Verification items for the finished model (mm, model axes). Face numbers are marked on the shaded views. A direction names the side the tool comes from. Coordinates: 2 decimals unless noted, no trailing zeros. Order: outer loops, then holes, each group sorted by start corner. A loop starts at its lowest first (then second) coordinate and runs counter-clockwise, first axis right, second up. Notation, with made-up numbers: M 53.5,-25.5 L 92.5,-25.5 A24 cw 92.5,-1.5 Z; hole C 57,-21.5 d2. An arc over 180 degrees is marked long. Return JSON: item names as keys, results as strings. Group by question number.
Q1. Section check C-C, the plane x = 33.8. Enter the section's corners in (y, z), then the cut area to 3 significant figures.
Q2. Thickness scan on probe 1 along Y at (x, z) = (33.8, 12); probe 2 along X at (y, z) = (64.8, 6.5); probe 3 along Y at (x, z) = (10, 4.25). Record the ranges inside material, lowest first.
Q3. Section check A-A, the plane z = 13.25. Count the separate pieces of the cut face and the enclosed holes in it, then the cut area to 3 significant figures.
Q4. Go/stop test with flat-tipped pins: pin 1 Ø4 at (x, y) = (25, 21.5) entering from -Z; pin 2 Ø5 at (x, y) = (9.5, 39.5) entering from +Z; pin 3 Ø1.3 at (x, y) = (10.5, 3.5) entering from +Z; pin 4 Ø2.5 at (x, z) = (17.5, 6) entering from +Y. Record where each tip stops, or that it passes through.
Q5. Section check B-B, the plane y = 48. Enter the section's corners in (x, z), then the cut area to 3 significant figures.
Q6. Access from +Z, -Z, +X, -X, +Y, -Y to the whole of each face (thin tool, end or side, straight path). Record for the marked faces 1, 2, 3, 4 and 5.
from build123d import *

# Parameters (mm, degrees)
SKETCH_W      = 36
SKETCH_H      = 67
PAD_DEPTH     = 2
SKETCH002_W   = 1.5
SKETCH002_H   = 22
SKETCH002_W_2 = 6
SKETCH002_H_2 = 1.5
PAD001_DEPTH  = 12.75
SKETCH001_W   = 21
SKETCH001_H   = 15
SKETCH001_R   = 0.8
PAD006_DEPTH  = 8
SKETCH018_W   = 4.4
SKETCH018_H   = 4.4
SKETCH018_R   = 0.8
PAD020_DEPTH  = 13.75


with BuildPart() as part:
    # Sketch → Pad (new body)
    with BuildSketch(Plane.XY):
        with Locations((18, 33.5)):
            Rectangle(SKETCH_W, SKETCH_H)
    extrude(amount=PAD_DEPTH)

    # Sketch002 (on DatumPlane) → Pad001 (join)
    with BuildSketch(Plane.XY.offset(2)):
        with Locations((10.25, 39.5)):
            Rectangle(SKETCH002_W, SKETCH002_H)
        with Locations((18, 29.25)):
            Rectangle(SKETCH002_W_2, SKETCH002_H_2)
        with Locations((25.75, 39.5)):
            Rectangle(SKETCH002_W, SKETCH002_H)
        with Locations((18, 49.75)):
            Rectangle(SKETCH002_W_2, SKETCH002_H_2)
    extrude(amount=PAD001_DEPTH)

    # Sketch001 (on DatumPlane) → Pad006 (join)
    with BuildSketch(Plane.XY.offset(2)):
        with Locations((18, 7.5)):
            Rectangle(SKETCH001_W, SKETCH001_H)
        with Locations((10.253, 3.69)):
            Circle(SKETCH001_R, mode=Mode.SUBTRACT)
        with Locations((25.747, 3.69)):
            Circle(SKETCH001_R, mode=Mode.SUBTRACT)
    extrude(amount=PAD006_DEPTH)

    # Sketch018 (on DatumPlane) → Pad020 (join)
    with BuildSketch(Plane.XY.offset(2)):
        with Locations((2.2, 2.2)):
            Rectangle(SKETCH018_W, SKETCH018_H)
        with Locations((2.2, 2.2)):
            Circle(SKETCH018_R, mode=Mode.SUBTRACT)
        with Locations((33.8, 2.2)):
            Rectangle(SKETCH018_W, SKETCH018_H)
        with Locations((33.8, 2.2)):
            Circle(SKETCH018_R, mode=Mode.SUBTRACT)
        with Locations((33.8, 64.8)):
            Rectangle(SKETCH018_W, SKETCH018_H)
        with Locations((33.8, 64.8)):
            Circle(SKETCH018_R, mode=Mode.SUBTRACT)
        with Locations((2.2, 64.8)):
            Rectangle(SKETCH018_W, SKETCH018_H)
        with Locations((2.2, 64.8)):
            Circle(SKETCH018_R, mode=Mode.SUBTRACT)
    extrude(amount=PAD020_DEPTH)


solid = part.part
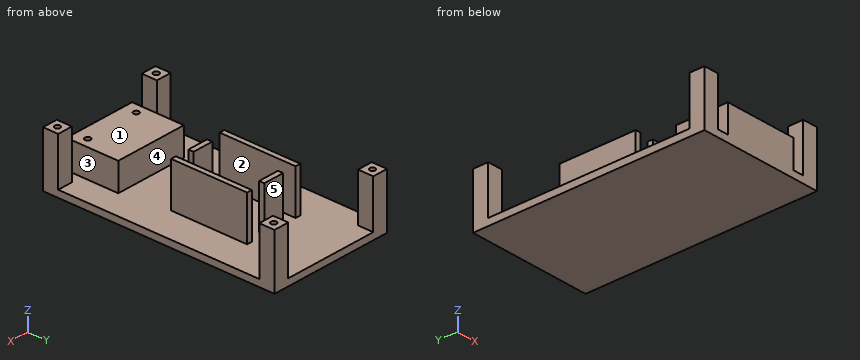
Numbers:
{
 "1": {"outline": "M 0,0 L 67,0 L 67,15.75 L 65.6,15.75 L 65.6,2 L 64,2 L 64,15.75 L 62.6,15.75 L 62.6,2 L 4.4,2 L 4.4,15.75 L 3,15.75 L 3,2 L 1.4,2 L 1.4,15.75 L 0,15.75 Z", "area": "211 mm2"},
 "2": {"probe 1": "y = 0 to 1.4, 3 to 4.4, 62.6 to 64, 65.6 to 67", "probe 2": "x = 0 to 1.4, 3 to 4.4, 31.6 to 33, 34.6 to 36", "probe 3": "y = 0 to 2.93, 4.45 to 15, 28.5 to 50.5"},
 "3": {"separate pieces": "8", "enclosed holes": "4", "area": "153 mm2"},
 "4": {"pin 1": "stops at z = 0", "pin 2": "stops at z = 14.75", "pin 3": "stops at z = 10", "pin 4": "stops at y = 50.5"},
 "5": {"outline": "M 0,0 L 36,0 L 36,2 L 26.5,2 L 26.5,14.75 L 25,14.75 L 25,2 L 11,2 L 11,14.75 L 9.5,14.75 L 9.5,2 L 0,2 Z", "area": "110 mm2"},
 "6": {"face 1": "+Z, -Y", "face 2": "+Z, +Y", "face 3": "+Z, +Y, -Y", "face 4": "+Z, +X, -X", "face 5": "+Z, +X, -X, +Y"}
}
